Read the model definition and answer for the solid it produces. Units are mm, in the model's axes. A direction names the side the tool comes from. Coordinates: 2 decimals unless noted, no trailing zeros. Write each loop counter-clockwise with the first axis right and the second up, starting at its lowest first coordinate (ties: lowest second). Pieces come first, ordered by that corner, then holes.
(1) Given pin 1 (3 mm diameter, centred on x = -2.5, z = -2, fed in from +Y); pin 2 (1.5 mm diameter, centred on x = -0.5, z = 9.5, fed in from +Y); pin 3 (12 mm diameter, centred on x = 7, z = 20.5, fed in from +Y); pin 4 (1.5 mm diameter, centred on x = -7, y = 36.5, fed in from +Z), each flat-ended and moving along its own axis, determine where each tip first touches the part or whether it passes through.
(2) Which of the six approach directions +Z, -Z, +X, -X, +Y, -Y give full straight-line access (tool end or side, diameter ignored) to faces 1 (the flat face through (0, 41, 9)), 2 (the flat face through (0, 0, 7)), 3 (the cylindrical face through (0.434, 40.493, -9.565))?
(3) Find the intervals of material crossed by probe 1 along Y at (x, z) = (-7, 3); probe 2 along Z at (x, y) = (-1.75, 33.5); probe 3 along Y at (x, z) = (-5, -6), in increasing order.
(4) Section D-D on z = 21 is taken. Write down the section's boundary in (x, y).
(5) Section C-C on y = 38.5 is taken. Write down the section's boundary in (x, z).
(6) Section A-A on z = 13 is taken. Write down the section's boundary in (x, y), then the cut area to 3 significant figures.
(7) Section B-B on x = 8.5 is taken. Write down the section's boundary in (y, z), then the cut area to 3 significant figures.
from build123d import *

# Parameters (mm, degrees)
SKETCH1_W           = 20
SKETCH1_H           = 41
BOSS_EXTRUDE1_DEPTH = 40
CHAMFER1_SIZE       = 10
SKETCH2_R           = 6
BOSS_EXTRUDE2_DEPTH = 2
FILLET1_R           = 1
SKETCH3_W           = 2.35715975
SKETCH3_H           = 15.320908912
BOSS_EXTRUDE3_DEPTH = 1
FILLET2_R           = 0.5
SKETCH4_R           = 3
BOSS_EXTRUDE4_DEPTH = 4
SKETCH5_R           = 0.2
CUT_EXTRUDE1_DEPTH  = 4


with BuildPart() as part:
    # Sketch1 → Boss-Extrude1 (new body)
    with BuildSketch(Plane(origin=(0, 0, 0), x_dir=(1, 0, 0), z_dir=(0, 1, 0))):
        with Locations((0, -6.919054605)):
            Rectangle(SKETCH1_W, SKETCH1_H)
    extrude(amount=BOSS_EXTRUDE1_DEPTH)

    # Chamfer1
    chamfer1_edges = [part.edges().sort_by_distance(p)[0] for p in [
        (0, 40, 27.419054605),
    ]]
    chamfer(chamfer1_edges, length=CHAMFER1_SIZE)

    # Sketch2 → Boss-Extrude2 (add)
    with BuildSketch(Plane(origin=(0, 40, 0), x_dir=(1, 0, 0), z_dir=(0, 1, 0))):
        with Locations(Location((0, 3.580945395, 0), (0, 0, 270))):
            Circle(SKETCH2_R)
    extrude(amount=BOSS_EXTRUDE2_DEPTH)

    # Fillet1
    fillet1_edges = [part.edges().sort_by_distance(p)[0] for p in [
        (0, 42, -9.580945395),
    ]]
    fillet(fillet1_edges, radius=FILLET1_R)

    # Sketch3 → Boss-Extrude3 (add)
    with BuildSketch(Plane(origin=(0, 40, 0), x_dir=(1, 0, 0), z_dir=(0, 1, 0))):
        with Locations((-0.179276882, -8.380978437)):
            Rectangle(SKETCH3_W, SKETCH3_H)
    extrude(amount=BOSS_EXTRUDE3_DEPTH)

    # Fillet2
    # the kernel refuses this fillet: 0.5 mm, written as the material it takes off along each edge
    with BuildSketch(Plane(origin=(0.999302993, 41, 1.085252162), x_dir=(-1, 0, 0), z_dir=(0, 0, 1))) as fillet2_piece_1_section:
        with BuildLine():
            CenterArc((FILLET2_R, FILLET2_R), FILLET2_R, 180, 90)
            Line((0, FILLET2_R), (0, 0))
            Line((0, 0), (FILLET2_R, 0))
        make_face()
    fillet2_piece_1 = extrude(amount=16.206180731, mode=Mode.PRIVATE)
    fillet2_piece_1 = fillet2_piece_1 - Plane(origin=(0, 40.888261374, -3.580945395), x_dir=(0, 0, 1), z_dir=(0, -1, 0)) * Cylinder(6, 35, mode=Mode.PRIVATE)
    add(fillet2_piece_1, mode=Mode.SUBTRACT)
    with BuildSketch(Plane(origin=(-1.357856757, 41, 17.291432893), x_dir=(1, 0, 0), z_dir=(0, 0, -1))) as fillet2_piece_2_section:
        with BuildLine():
            CenterArc((FILLET2_R, FILLET2_R), FILLET2_R, 180, 90)
            Line((0, FILLET2_R), (0, 0))
            Line((0, 0), (FILLET2_R, 0))
        make_face()
    fillet2_piece_2 = extrude(amount=16.27804556, mode=Mode.PRIVATE)
    fillet2_piece_2 = fillet2_piece_2 - Plane(origin=(0, 40.888238096, -3.580945395), x_dir=(0, 0, 1), z_dir=(0, -1, 0)) * Cylinder(6, 35, mode=Mode.PRIVATE)
    add(fillet2_piece_2, mode=Mode.SUBTRACT)
    with BuildSketch(Plane(origin=(2.249302993, 41, 16.041432893), x_dir=(0, 0, -1), z_dir=(-1, 0, 0))) as fillet2_piece_3:
        with BuildLine():
            CenterArc((FILLET2_R, FILLET2_R), FILLET2_R, 180, 90)
            Line((0, FILLET2_R), (0, 0))
            Line((0, 0), (FILLET2_R, 0))
        make_face()
    extrude(amount=4.85715975, mode=Mode.SUBTRACT)

    # Sketch4 → Boss-Extrude4 (add)
    with BuildSketch(Plane(origin=(0, 42, 0), x_dir=(1, 0, 0), z_dir=(0, 1, 0))):
        with Locations(Location((0, 3.580945395, 0), (0, 0, 270))):
            Circle(SKETCH4_R)
    extrude(amount=BOSS_EXTRUDE4_DEPTH)

    # Sketch5 → Cut-Extrude1 (cut)
    with BuildSketch(Plane(origin=(0, 46, 0), x_dir=(1, 0, 0), z_dir=(0, 1, 0))):
        with Locations((0, 0.580945395)):
            Circle(SKETCH5_R)
        with Locations((-0.375999701, 0.604601291)):
            Circle(SKETCH5_R)
        with Locations((-0.746069661, 0.675195911)):
            Circle(SKETCH5_R)
        with Locations((-1.104373658, 0.791615937)):
            Circle(SKETCH5_R)
        with Locations((-1.445261022, 0.952025355)):
            Circle(SKETCH5_R)
        with Locations((-1.763355757, 1.153894412)):
            Circle(SKETCH5_R)
        with Locations((-2.053641318, 1.394039512)):
            Circle(SKETCH5_R)
        with Locations((-2.311539728, 1.668673425)):
            Circle(SKETCH5_R)
        with Locations((-2.532983777, 1.97346501)):
            Circle(SKETCH5_R)
        with Locations((-2.714481157, 2.30360752)):
            Circle(SKETCH5_R)
        with Locations((-2.853169549, 2.653894412)):
            Circle(SKETCH5_R)
        with Locations((-2.946861752, 3.018801451)):
            Circle(SKETCH5_R)
        with Locations((-2.994080185, 3.392573836)):
            Circle(SKETCH5_R)
        with Locations((-2.994080185, 3.769316953)):
            Circle(SKETCH5_R)
        with Locations((-2.946861752, 4.143089338)):
            Circle(SKETCH5_R)
        with Locations((-2.853169549, 4.507996378)):
            Circle(SKETCH5_R)
        with Locations((-2.714481157, 4.858283269)):
            Circle(SKETCH5_R)
        with Locations((-2.532983777, 5.18842578)):
            Circle(SKETCH5_R)
        with Locations((-2.311539728, 5.493217364)):
            Circle(SKETCH5_R)
        with Locations((-2.053641318, 5.767851277)):
            Circle(SKETCH5_R)
        with Locations((-1.763355757, 6.007996378)):
            Circle(SKETCH5_R)
        with Locations((-1.445261022, 6.209865435)):
            Circle(SKETCH5_R)
        with Locations((-1.104373658, 6.370274852)):
            Circle(SKETCH5_R)
        with Locations((-0.746069661, 6.486694878)):
            Circle(SKETCH5_R)
        with Locations((-0.375999701, 6.557289499)):
            Circle(SKETCH5_R)
        with Locations((0, 6.580945395)):
            Circle(SKETCH5_R)
        with Locations((0.375999701, 6.557289499)):
            Circle(SKETCH5_R)
        with Locations((0.746069661, 6.486694878)):
            Circle(SKETCH5_R)
        with Locations((1.104373658, 6.370274852)):
            Circle(SKETCH5_R)
        with Locations((1.445261022, 6.209865435)):
            Circle(SKETCH5_R)
        with Locations((1.763355757, 6.007996378)):
            Circle(SKETCH5_R)
        with Locations((2.053641318, 5.767851277)):
            Circle(SKETCH5_R)
        with Locations((2.311539728, 5.493217364)):
            Circle(SKETCH5_R)
        with Locations((2.532983777, 5.18842578)):
            Circle(SKETCH5_R)
        with Locations((2.714481157, 4.858283269)):
            Circle(SKETCH5_R)
        with Locations((2.853169549, 4.507996378)):
            Circle(SKETCH5_R)
        with Locations((2.946861752, 4.143089338)):
            Circle(SKETCH5_R)
        with Locations((2.994080185, 3.769316953)):
            Circle(SKETCH5_R)
        with Locations((2.994080185, 3.392573836)):
            Circle(SKETCH5_R)
        with Locations((2.946861752, 3.018801451)):
            Circle(SKETCH5_R)
        with Locations((2.853169549, 2.653894412)):
            Circle(SKETCH5_R)
        with Locations((2.714481157, 2.30360752)):
            Circle(SKETCH5_R)
        with Locations((2.532983777, 1.97346501)):
            Circle(SKETCH5_R)
        with Locations((2.311539728, 1.668673425)):
            Circle(SKETCH5_R)
        with Locations((2.053641318, 1.394039512)):
            Circle(SKETCH5_R)
        with Locations((1.763355757, 1.153894412)):
            Circle(SKETCH5_R)
        with Locations((1.445261022, 0.952025355)):
            Circle(SKETCH5_R)
        with Locations((1.104373658, 0.791615937)):
            Circle(SKETCH5_R)
        with Locations((0.746069661, 0.675195911)):
            Circle(SKETCH5_R)
        with Locations((0.375999701, 0.604601291)):
            Circle(SKETCH5_R)
    extrude(amount=-CUT_EXTRUDE1_DEPTH, mode=Mode.SUBTRACT)


solid = part.part
Response:
1. pin 1: stops at y = 46
1. pin 2: stops at y = 41
1. pin 3: stops at y = 40
1. pin 4: stops at z = 21.67
2. face 1: +Z, +X, -X, +Y
2. face 2: +Z, -Z, +X, -X, -Y
2. face 3: +Y
3. probe 1: y = 0 to 40
3. probe 2: z = -13.58 to 23.92
3. probe 3: y = 0 to 41.83
4. outline: (-10, 0) - (10, 0) - (10, 36.42) - (-10, 36.42) - close
5. outline: (-10, -13.58) - (10, -13.58) - (10, 18.92) - (-10, 18.92) - close
6. outline: (-10, 0) - (10, 0) - (10, 40) - (1, 40) - (1, 40.5) arc R0.5 ccw to (0.5, 41) - (-0.86, 41) arc R0.5 ccw to (-1.36, 40.5) - (-1.36, 40) - (-10, 40) - close
6. area: 802 mm2
7. outline: (0, -13.58) - (40, -13.58) - (40, 17.42) - (30, 27.42) - (0, 27.42) - close
7. area: 1,590 mm2
